```python
from build123d import *

# Parameters (mm, degrees)
SALIENTE_EXTRUIR1_START = 2
SALIENTE_EXTRUIR1_DEPTH = 5
CROQUIS2_W              = 30
CROQUIS2_H              = 25
SALIENTE_EXTRUIR2_DEPTH = 2
CROQUIS3_R              = 1.5
CORTAR_EXTRUIR1_DEPTH   = 10
CROQUIS4_R              = 1.500036904
CROQUIS4_R_2            = 1.5
CORTAR_EXTRUIR2_DEPTH   = 10
CROQUIS6_W              = 5
CROQUIS6_H              = 55
SALIENTE_EXTRUIR3_DEPTH = 15
CROQUIS7_R              = 1.5
CORTAR_EXTRUIR3_DEPTH   = 20


with BuildPart() as part:
    # Croquis1 → Saliente-Extruir1 (new body)
    with BuildSketch(Plane.XY.offset(SALIENTE_EXTRUIR1_START)):
        Polygon((65.454041039, -1015), (65.454041039, -1005), (95.454041039, -1005), (95.454041039, -1015), (95.454041039, -1105), (65.454041039, -1105), align=None)
    extrude(amount=SALIENTE_EXTRUIR1_DEPTH)

    # Croquis2 → Saliente-Extruir2 (add)
    with BuildSketch(Plane(origin=(0, 0, 2), x_dir=(-1, 0, 0), z_dir=(0, 0, -1))):
        with Locations((-80.454041039, -1017.5)):
            Rectangle(CROQUIS2_W, CROQUIS2_H)
    extrude(amount=SALIENTE_EXTRUIR2_DEPTH)

    # Croquis3 → Cortar-Extruir1 (cut)
    with BuildSketch(Plane(origin=(0, 0, 2), x_dir=(-1, 0, 0), z_dir=(0, 0, -1))):
        with Locations((-72.954041039, -1070)):
            Circle(CROQUIS3_R)
        with Locations((-87.954041039, -1095)):
            Circle(CROQUIS3_R)
    extrude(amount=-CORTAR_EXTRUIR1_DEPTH, mode=Mode.SUBTRACT)

    # Croquis4 → Cortar-Extruir2 (cut)
    with BuildSketch(Plane(origin=(0, 0, 0), x_dir=(-1, 0, 0), z_dir=(0, 0, -1))):
        with Locations((-92.454041038, -1014.999963096)):
            Circle(CROQUIS4_R)
        with Locations((-68.454041039, -1015)):
            Circle(CROQUIS4_R_2)
    extrude(amount=-CORTAR_EXTRUIR2_DEPTH, mode=Mode.SUBTRACT)

    # Croquis6 → Saliente-Extruir3 (add)
    with BuildSketch(Plane(origin=(95.454041039, 0, 0), x_dir=(0, 0, -1), z_dir=(1, 0, 0))):
        with Locations((-4.5, -1032.456092312)):
            Rectangle(CROQUIS6_W, CROQUIS6_H)
    extrude(amount=SALIENTE_EXTRUIR3_DEPTH)

    # Croquis7 → Cortar-Extruir3 (cut)
    with BuildSketch(Plane.XY.offset(7)):
        with Locations((102.954041039, -1051.956092312)):
            Circle(CROQUIS7_R)
        with Locations((102.954041039, -1021.956092312)):
            Circle(CROQUIS7_R)
    extrude(amount=-CORTAR_EXTRUIR3_DEPTH, mode=Mode.SUBTRACT)


solid = part.part
```
The model under review builds one solid part; all positions refer to its coordinate system, in mm. A direction names the side the tool comes from. Coordinates: 2 decimals unless noted, no trailing zeros. Order: outer loops, then holes, each group sorted by start corner. A loop starts at its lowest first (then second) coordinate and runs counter-clockwise, first axis right, second up. Notation, with made-up numbers: (-23, 14.5) -> (28, 14.5) arc R30 ccw to (28, 39.5) -> close; hole circle Ø10 at (64, 76.5). An arc over 180 degrees is marked (long way). Answer in a Markdown table with one row per item. Add a question column.
Item 1: We need section C-C on x = 83. Write out the cut boundary in (y, z), plus the area to 3 significant figures.
Item 2: Clearance check with flat-ended pins moving along their axes: pin 1 (4 mm diameter, centred on y = -1083.5, z = 5.5, fed in from +X); pin 2 (1.8 mm diameter, centred on x = 72.95, y = -1070, fed in from +Z); pin 3 (2 mm diameter, centred on x = 74.5, z = 5, fed in from +Y); pin 4 (22.5 mm diameter, centred on x = 97, y = -1043, fed in from -Z). State where each tip first meets the part, or that it passes through.
Item 3: To check wall thickness, follow probe 1 along X at (y, z) = (-1095, 3.65); probe 2 along Z at (x, y) = (106, -1021.5); probe 3 along X at (y, z) = (-1053, 3.25). State the ranges of each line that lie inside material, in increasing order.
Item 4: We need section B-B on z = 4.25. Write out the cut boundary in (x, y).
Item 5: We need section D-D on y = -1046.5. Write out the cut boundary in (x, z).
Item 6: We need section A-A on y = -1095. Write out the cut boundary in (x, z).
Item 7: Mouldability with a two-part tool opening along Y and no side actions: class faces 1 (the flat face through (81, -1005, 4)), 2 (the cylindrical face through (101.85, -1050.94, 4.54)), 3 (the flat face through (110.454, -1032, 5)) as +Y half, -Y half, draft (parallel to the pull), parting line (faces both ways), or undercut.
Item 8: Machinability: for faces 4 (the flat face through (103, -1004.956, 5)), 5 (the flat face through (95.454, -1083, 5)), 6 (the flat face through (81, -1030, 1)), 7 (the cylindrical face through (68.649, -1013.513, 3.451)), 8 (the flat face through (95.454, -1018, 1)), which of the approach directions +Z, -Z, +X, -X, +Y, -Y give a long, thin tool a straight path to every point of the face, cutting with its end or side? Answer none if there is none.
Final values:
| question | item | result |
|---|---|---|
| 1 | outline | (-1105, 2) -> (-1030, 2) -> (-1030, 0) -> (-1005, 0) -> (-1005, 7) -> (-1105, 7) -> close |
| 1 | area | 550 mm2 |
| 2 | pin 1 | stops at x = 95.45 |
| 2 | pin 2 | passes through |
| 2 | pin 3 | stops at y = -1005 |
| 2 | pin 4 | stops at z = 2 |
| 3 | probe 1 | x = 65.45 to 86.45, 89.45 to 95.45 |
| 3 | probe 2 | z = 2 to 7 |
| 3 | probe 3 | x = 65.45 to 101.88, 104.03 to 110.45 |
| 4 | outline | (65.45, -1105) -> (95.45, -1105) -> (95.45, -1059.96) -> (110.45, -1059.96) -> (110.45, -1004.96) -> (95.45, -1004.96) -> (95.45, -1005) -> (65.45, -1005) -> close; hole circle Ø3 at (68.45, -1015); hole circle Ø3 at (72.95, -1070); hole circle Ø3 at (87.95, -1095); hole circle Ø3 at (92.45, -1015); hole circle Ø3 at (102.95, -1051.96); hole circle Ø3 at (102.95, -1021.96) |
| 5 | outline | (65.45, 2) -> (110.45, 2) -> (110.45, 7) -> (65.45, 7) -> close |
| 6 | outline | (65.45, 2) -> (86.45, 2) -> (86.45, 7) -> (65.45, 7) -> close; (89.45, 2) -> (95.45, 2) -> (95.45, 7) -> (89.45, 7) -> close |
| 7 | face 1 | +Y half |
| 7 | face 2 | undercut |
| 7 | face 3 | draft |
| 8 | face 4 | +Z, -Z, +X, -X, +Y |
| 8 | face 5 | +Z, -Z, +X, -Y |
| 8 | face 6 | -Z, +X, -X, -Y |
| 8 | face 7 | +Z, -Z |
| 8 | face 8 | -Z, +X, +Y, -Y |
